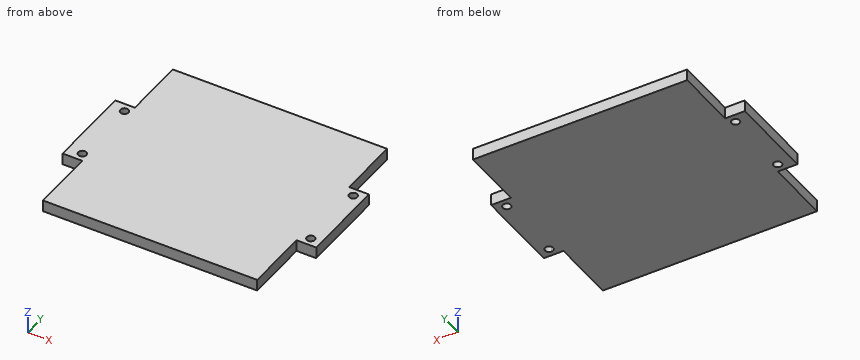
from build123d import *

# Parameters (mm, degrees)
F0_R     = 1.75
F1_DEPTH = 5


with BuildPart() as f1:
    # F0 (on Top) → F1 (new body)
    with BuildSketch(Plane.XY):
        with BuildLine():
            Line((57.7837471709, 69.5580622628), (-34.7162528291, 69.5580622628))
            Line((-34.7162528291, 69.5580622628), (-34.7162528291, 42.5580622628))
            Line((-34.7162528291, 42.5580622628), (-43.2162528291, 42.5580622628))
            Line((-43.2162528291, 42.5580622628), (-43.2162528291, 5.0580622628))
            Line((-43.2162528291, 5.0580622628), (-34.7162528291, 5.0580622628))
            Line((-34.7162528291, 5.0580622628), (-34.7162528291, -22.9419377372))
            Line((-34.7162528291, -22.9419377372), (57.7837471709, -22.9419377372))
            Line((57.7837471709, -22.9419377372), (57.7837471709, 5.0580622628))
            Line((57.7837471709, 5.0580622628), (61.776727438, 5.0580622628))
            Line((61.776727438, 5.0580622628), (61.7764500569, 6.9623562581))
            ThreePointArc((61.7764500569, 6.9623562581), (60.5385780505, 9.9496128474), (63.5261951319, 8.712611146))
            Line((63.5261951319, 8.712611146), (66.3054800854, 8.713015979))
            Line((66.3054800854, 8.713015979), (66.3054800854, 42.5580622628))
            Line((66.3054800854, 42.5580622628), (57.7837471709, 42.5580622628))
            Line((57.7837471709, 42.5580622628), (57.7837471709, 69.5580622628))
        make_face()
        with Locations((-36.9397651508, 8.7772880495)):
            Circle(F0_R, mode=Mode.SUBTRACT)
        with Locations((-36.9361157864, 38.7772880495)):
            Circle(F0_R, mode=Mode.SUBTRACT)
        with Locations((61.7687867672, 38.9017461427)):
            Circle(F0_R, mode=Mode.SUBTRACT)
        with BuildLine():
            Line((66.3054800854, 5.0580622628), (66.3054800854, 8.713015979))
            Line((66.3054800854, 8.713015979), (63.5261951319, 8.712611146))
            ThreePointArc((63.5261951319, 8.712611146), (63.5261951458, 8.7124836928), (63.5261951505, 8.7123562396))
            ThreePointArc((63.5261951505, 8.7123562396), (63.0137221373, 7.4750094988), (61.7764500569, 6.9623562581))
            Line((61.7764500569, 6.9623562581), (61.776727438, 5.0580622628))
            Line((61.776727438, 5.0580622628), (66.3054800854, 5.0580622628))
        make_face()
    extrude(amount=F1_DEPTH)


solid = f1.part
Build history of the part. All positions in model axes, mm. Round coordinates to 2 decimals unless told otherwise and drop trailing zeros. Order: outer loops, then holes, each group sorted by start corner. A loop starts at its lowest first (then second) coordinate and runs counter-clockwise, first axis right, second up. Notation, with made-up numbers: M -5,-5 L 25,-5 A13 ccw 25,0 Z; hole C 51,-15.75 d5. An arc over 180 degrees is marked long. Use CSV: the item, a comma, the result in double quotes. Start each with the question number.
(1) Flat gauge pins, fed straight in: P1, Ø2.5, axis at y = -3, z = 1.5, coming from the +X side; P2, Ø1.5, axis at y = -14.5, z = 1.5, coming from the -X side; P3, Ø1.5, axis at x = -40, z = 2.5, coming from the +Y side. Where does each tip first touch, or does it go through?
(2) Cut at A-A on z = 3.2. State how many separate pieces and enclosed holes the cut face has, then the cut area to 3 significant figures.
(3) Drill centre lines: probe 1 along X at (y, z) = (8.5, 3.5); probe 2 along X at (y, z) = (9, 3.5); probe 3 along X at (y, z) = (5, 0.25). Where is each one in solid material? Low to high.
(4) Cut at B-B on y = 50.5. List the corners of the cut face in (x, z), then the cut area to 4 significant figures.
Findings:
1,P1,"stops at x = 57.78"
1,P2,"stops at x = -34.72"
1,P3,"stops at y = 42.56"
2,separate pieces,"1"
2,enclosed holes,"4"
2,area,"9,160 mm^2"
3,probe 1,"x = -43.22 to -38.67, -35.21 to 60.04, 63.51 to 66.31"
3,probe 2,"x = -43.22 to -38.68, -35.2 to 60.05, 63.5 to 66.31"
3,probe 3,"x = -34.72 to 57.78"
4,outline,"M -34.72,0 L 57.78,0 L 57.78,5 L -34.72,5 Z"
4,area,"462.5 mm^2"
